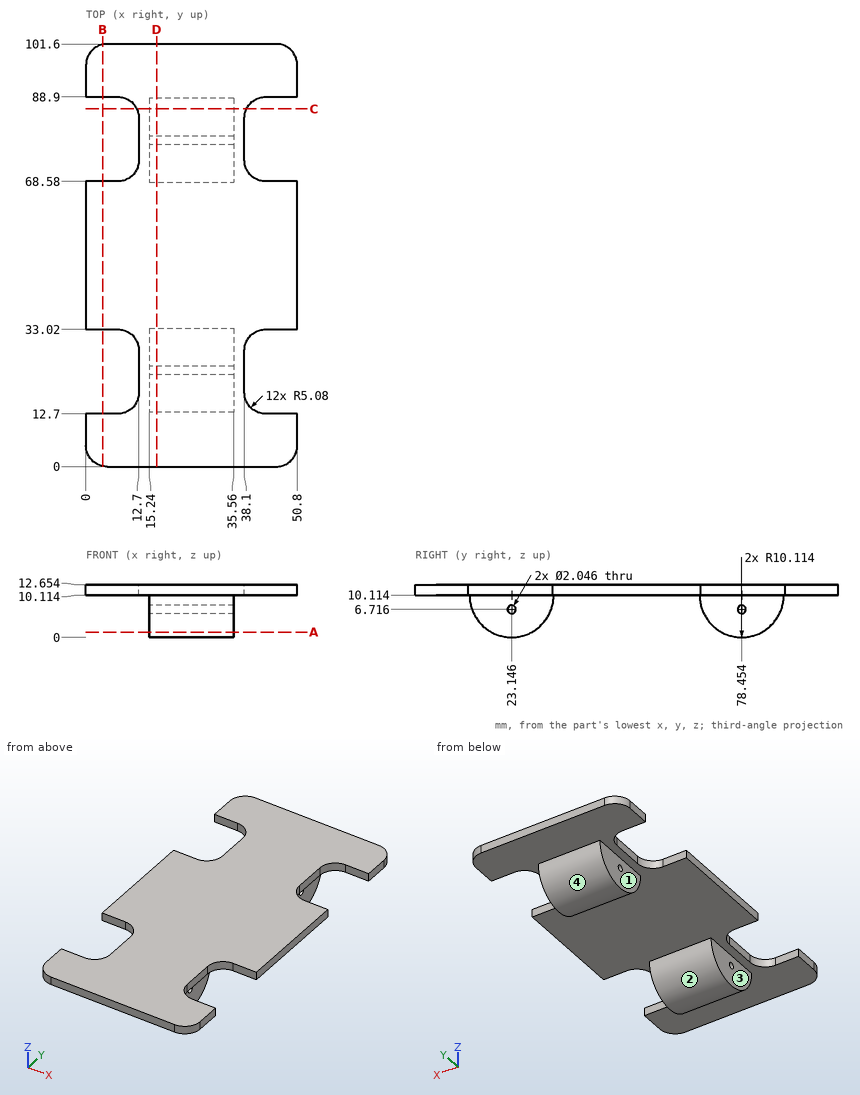
Design review of the part shown in the three views and the two pictorial views. Dimensions are in mm from the part's minimum x, y and z. A direction names the side the tool comes from. Give positions to 0.01 mm unless a question says otherwise; leave off trailing zeros. Loops run counter-clockwise (first coordinate to the right, second up) from the corner with the lowest first, then second, coordinate; pieces in that order, holes last. Notation, with made-up numbers: (1.5, 27) - (9.5, 27) arc R17 ccw to (9.5, 39) - close; hole circle Ø8 at (36, 24). An arc over 180 degrees is marked (long way). Answer as a JSON object with one key per item and string values.
Q1. Add section B-B on x = 4. State the section outline as (y, z) points (1 decimal), plus the area to 3 significant figures.
Worked out:
{"outline": "(0.1, 10.1) - (12.7, 10.1) - (12.7, 12.7) - (0.1, 12.7) - close; (33, 10.1) - (68.6, 10.1) - (68.6, 12.7) - (33, 12.7) - close; (88.9, 10.1) - (101.5, 10.1) - (101.5, 12.7) - (88.9, 12.7) - close", "area": "154 mm^2"}
Q2. Add section A-A on z = 1.25. State the section outline as (x, y) points (1 decimal), plus the area to 3 significant figures.
Worked out:
{"outline": "(15.2, 18.3) - (35.6, 18.3) - (35.6, 28) - (15.2, 28) - close; (15.2, 73.6) - (35.6, 73.6) - (35.6, 83.3) - (15.2, 83.3) - close", "area": "396 mm^2"}
Q3. Mouldability with a two-part tool opening along Y and no side actions: class the marked faces 1 and 2 as +Y half, -Y half, draft (parallel to the pull), parting line (faces both ways), or undercut.
Worked out:
{"face 1": "draft", "face 2": "undercut"}
Q4. For the marked faces 3 and 4, list the 3-axis set-ups (+Z, -Z, +X, -X, +Y, -Y) from which the entire face can be reached by the end or side of a thin tool; tool diameter is ignored.
Worked out:
{"face 3": "-Z, -X, +Y, -Y", "face 4": "-Z, +X, -X"}
Q5. Add section D-D on x = 17. State the section outline as (y, z) points (1 decimal).
Worked out:
{"outline": "(0, 10.1) - (13, 10.1) arc R10.1 ccw to (33.3, 10.1) - (68.3, 10.1) arc R10.1 ccw to (88.6, 10.1) - (101.6, 10.1) - (101.6, 12.7) - (0, 12.7) - close; hole circle Ø2 at (23.1, 6.7); hole circle Ø2 at (78.5, 6.7)"}
Q6. Add section C-C on y = 86. State the section outline as (x, z) points (1 decimal), plus the area to 3 significant figures.
Worked out:
{"outline": "(12.2, 10.1) - (15.2, 10.1) - (15.2, 3.4) - (35.6, 3.4) - (35.6, 10.1) - (38.6, 10.1) - (38.6, 12.7) - (12.2, 12.7) - close", "area": "204 mm^2"}
Q7. Insertion check: pin 1 (1.5 mm diameter, centred on x = 28.5, z = 4.5, fed in from +Y); pin 2 (3.5 mm diameter, centred on y = 78.45, z = 6.72, fed in from -X); pin 3 (3 mm diameter, centred on y = 76.5, z = 11, fed in from -X); pin 4 (1.6 mm diameter, centred on y = 23.15, z = 6.72, fed in from +X). Each pin has a flat end and moves straight along its axis. Give the tip position at first contact, or say it passes through.
Worked out:
{"pin 1": "stops at y = 87.32", "pin 2": "stops at x = 15.24", "pin 3": "stops at x = 12.7", "pin 4": "passes through"}
Q8. To check wall thickness, follow line 1 along Y through (x, z) = (6, 11); line 2 along Y through (x, z) = (29, 10); line 3 along Z through (x, y) = (24, 56) (1 decimal). State the ranges of each line that lie inside material, in increasing order.
Worked out:
{"line 1": "y = 0 to 12.7, 33.02 to 68.58, 88.9 to 101.6", "line 2": "y = 13.03 to 33.26, 68.34 to 88.57", "line 3": "z = 10.1 to 12.7"}
